The listing builds one solid part. Answer for the finished solid, in the listing's coordinates (mm). A direction names the side the tool comes from. Coordinates: 2 decimals unless noted, no trailing zeros. Order: outer loops, then holes, each group sorted by start corner. A loop starts at its lowest first (then second) coordinate and runs counter-clockwise, first axis right, second up. Notation, with made-up numbers: (81, 4) -> (104, 4) arc R33 ccw to (104, 35) -> close; hole circle Ø10 at (-35.5, 13.5). An arc over 180 degrees is marked (long way). One line per question, with ' | ' between items.
from build123d import *

# Parameters (mm, degrees)
F0_W           = 40.25
F0_H           = 40.25
F1_DEPTH       = 56.45
F2_W           = 33.9
F2_H           = 33.9
F3_DEPTH       = 28
F5_D           = 11
F5_CBORE_D     = 17.25
F5_CBORE_DEPTH = 10
F6_SIZE2       = 11.849251
F6_SIZE        = 3.17499
F8_W           = 4.7625
F8_H           = 17.4625
F9_DEPTH       = 40.251
F10_SIZE       = 0.5


# Not quite as in the source:
# - a fillet or chamfer is up to 0.001 mm smaller than in the source, because OpenCascade refuses the exact size


with BuildPart() as f1:
    # F0 (on Top) → F1 (new body)
    with BuildSketch(Plane.XY):
        Rectangle(F0_W, F0_H)
    extrude(amount=F1_DEPTH)

    # F2 (on face) → F3 (cut)
    with BuildSketch(Plane.XY.offset(56.45)):
        Rectangle(F2_W, F2_H)
    extrude(amount=-F3_DEPTH, mode=Mode.SUBTRACT)

    # F5 (through all)
    with Locations(Plane.XY.offset(28.45)):
        with Locations((0, 0)):
            CounterBoreHole(F5_D / 2, F5_CBORE_D / 2, F5_CBORE_DEPTH)

    # F6 (size 3.175 and 11.849261314 in the source; OpenCascade refuses exactly that, so slightly less here)
    f6_edges = [f1.edges().sort_by_distance(p)[0] for p in [
        (0, 20.125, 56.45),
        (20.125, 0, 56.45),
        (0, -20.125, 56.45),
        (-20.125, 0, 56.45),
    ]]
    f6_side = f1.faces().sort_by_distance((0, -19.555779, 56.45))[0]
    chamfer(f6_edges, length=F6_SIZE, length2=F6_SIZE2, reference=f6_side)

    # F8 (on offset) → F9 (cut, through all)
    with BuildSketch(Plane(origin=(0, 20.125, 0), x_dir=(-1, 0, 0), z_dir=(0, 1, 0))):
        with BuildLine():
            ThreePointArc((-2.38125, 34.00625), (0, 31.625), (2.38125, 34.00625))
            Line((2.38125, 34.00625), (-2.38125, 34.00625))
        make_face()
        with Locations((0, 42.7375)):
            Rectangle(F8_W, F8_H)
        with BuildLine():
            Line((-2.38125, 51.46875), (2.38125, 51.46875))
            ThreePointArc((2.38125, 51.46875), (0, 53.85), (-2.38125, 51.46875))
        make_face()
    extrude(amount=-F9_DEPTH, mode=Mode.SUBTRACT)

    # F10
    f10_edges = [f1.edges().sort_by_distance(p)[0] for p in [
        (20.125, 0, 0),
        (0, -20.125, 0),
        (-20.125, 0, 0),
        (0, 20.125, 0),
    ]]
    chamfer(f10_edges, length=F10_SIZE)


solid = f1.part
Item 1: Section B-B, the plane x = 0 is taken. Count the separate pieces of the cut face and the enclosed holes in it, plus the area to 3 significant figures.
Computed values:
separate pieces: 4 | enclosed holes: 0 | area: 791 mm^2
Item 2: Section C-C, the plane z = 15.5 is taken. Give the vertices of the cut face in (x, y) (3 decimals), plus the area to 3 significant figures.
Computed values:
outline: (-20.125, -20.125) -> (20.125, -20.125) -> (20.125, 20.125) -> (-20.125, 20.125) -> close; hole circle Ø11 at (0, 0) | area: 1,530 mm^2
Item 3: Find the intervals of material crossed by L1, parallel to Y at x = 0, z = 5.75 (3 decimals); L2, parallel to Y at x = 7.5, z = 44 (3 decimals); L3, parallel to Z at x = 3.5, y = -6.5, in increasing order.
Computed values:
L1: y = -20.125 to -5.5, 5.5 to 20.125 | L2: y = -20.125 to -16.95, 16.95 to 20.125 | L3: z = 0 to 18.45
Item 4: For faces 5 (the face through (-18.56, -0.28, 50.44)), 6 (the face through (-2.381, -19, 43)), 7 (the face through (4, -16.95, 43)), determine the directions among +Z, -Z, +X, -X, +Y, -Y from which every point of the face is accessible in a straight line to the end or side of a thin tool.
Computed values:
face 5: +Z, -X, +Y, -Y | face 6: +Y, -Y | face 7: +Z
Item 5: Determine the mould class of faces 1 (the face through (-2.381, 19, 43)), 2 (the face through (4.19, -18.56, 50.44)), 3 (the face through (8.227, 2.591, 23.52)), 4 (the face through (-16.95, 0, 43)) for opening direction Y: pulls with the +Y half, pulls with the -Y half, needs draft (parallel to the pull), parting line crosses it, or undercut.
Computed values:
face 1: needs draft | face 2: pulls with the -Y half | face 3: undercut | face 4: undercut
Item 6: Each of these flat-tipped pins is pushed along its axis until it touches: pin 1 Ø14 at (x, z) = (7, 49) entering from -Y (3 decimals); pin 2 Ø17 at (x, y) = (-6, -0.5) entering from +Z; pin 3 Ø1 at (y, z) = (19, 46) entering from +X; pin 4 Ø5 at (x, y) = (5.5, -16) entering from +Z. Where does it stop, or does it pass through?
Computed values:
pin 1: stops at y = -20.125 | pin 2: stops at z = 28.45 | pin 3: stops at x = 19.88 | pin 4: stops at z = 56.45
